Can you work these out from the model? Positions are in its coordinate system, mm. Face numbers are marked on the shaded views. A direction names the side the tool comes from. Give positions to 0.01 mm unless a question says otherwise; leave off trailing zeros. Loops run counter-clockwise (first coordinate to the right, second up) from the corner with the lowest first, then second, coordinate; pieces in that order, holes last. Notation, with made-up numbers: (74.5, 66.5) - (89.5, 66.5) arc R16 ccw to (89.5, 92.5) - close; hole circle Ø4 at (20, 23). An arc over 180 degrees is marked (long way). Answer as a JSON object with one key per item and string values. Group by question number.
Item 1: Thinking about a two-plate mould opening in X: for the marked faces 6, 7 and 8, which applies, pulls with the +X half, pulls with the -X half, needs draft (parallel to the pull), parting line crosses it, or undercut?
Item 2: Please list where these lines run through material, in increasing order: L1, parallel to X at y = 7.5, z = 3; L2, parallel to X at y = 11.5, z = -4; L3, parallel to Y at x = -13.5, z = 2.75.
Item 3: Suppose I cut it at A-A on z = 0. Count the separate pieces of the cut face and the enclosed holes in it, and give its area (3 significant figures).
Item 4: Suppose I cut it at B-B on y = 8.5. Write out the boundary of the cut face in (x, z), and give its area (3 significant figures).
Item 5: Which directions (+Z, -Z, +X, -X, +Y, -Y) give clear straight access to the entire face, cutting with the end or side of a thin tool? Please do the marked faces 1, 2, 3, 4 and 5.
Item 6: Will these pins go through, and if not, where does the flat tip stop? pin 1 (3.5 mm diameter, centred on x = 27.24, z = 0, fed in from -Y); pin 2 (3 mm diameter, centred on y = 6.5, z = -1.5, fed in from +X); pin 3 (3 mm diameter, centred on y = 6.5, z = 0, fed in from -X).
Item 7: Suppose I cut it at C-C on x = 26.5. Write out the boundary of the cut face in (y, z).
from build123d import *

# Parameters (mm, degrees)
BOSS_EXTRUDE1_DEPTH = 4.7625
FILLET1_R           = 1.5875
FILLET2_R           = 3.175
FILLET3_R           = 3.175
HOLE1_D             = 2.8448
HOLE2_D             = 2.8448


with BuildPart() as part:
    # Sketch1 → Boss-Extrude1 (new body, symmetric)
    with BuildSketch(Plane.XY):
        Polygon((-29.1465, 11.1125), (-16.764, 11.1125), (-16.764, 0), (16.764, 0), (16.764, 11.1125), (37.9095, 11.1125), (37.9095, 12.7), (15.1765, 12.7), (15.1765, 1.5875), (-15.1765, 1.5875), (-15.1765, 12.7), (-29.1465, 12.7), align=None)
    extrude(amount=BOSS_EXTRUDE1_DEPTH, both=True)

    # Fillet1
    fillet1_edges = [part.edges().sort_by_distance(p)[0] for p in [
        (-15.1765, 1.5875, 0),
        (15.1765, 1.5875, 0),
        (16.764, 11.1125, 0),
        (-16.764, 11.1125, 0),
    ]]
    fillet(fillet1_edges, radius=FILLET1_R)

    # Fillet2
    fillet2_edges = [part.edges().sort_by_distance(p)[0] for p in [
        (-15.1765, 12.7, 0),
        (15.1765, 12.7, 0),
        (16.764, 0, 0),
        (-16.764, 0, 0),
    ]]
    fillet(fillet2_edges, radius=FILLET2_R)

    # Fillet3
    fillet3_edges = [part.edges().sort_by_distance(p)[0] for p in [
        (37.9095, 11.90625, -4.7625),
        (-29.1465, 11.90625, -4.7625),
        (37.9095, 11.90625, 4.7625),
        (-29.1465, 11.90625, 4.7625),
    ]]
    fillet(fillet3_edges, radius=FILLET3_R)

    # Hole1 (through all)
    with Locations(Plane.XZ.offset(-11.1125)):
        with Locations((27.2415, 0)):
            Hole(HOLE1_D / 2)

    # Hole2 (through all)
    with Locations(Plane.XZ.offset(-11.1125)):
        with Locations((-23.5585, 0)):
            Hole(HOLE2_D / 2)


solid = part.part
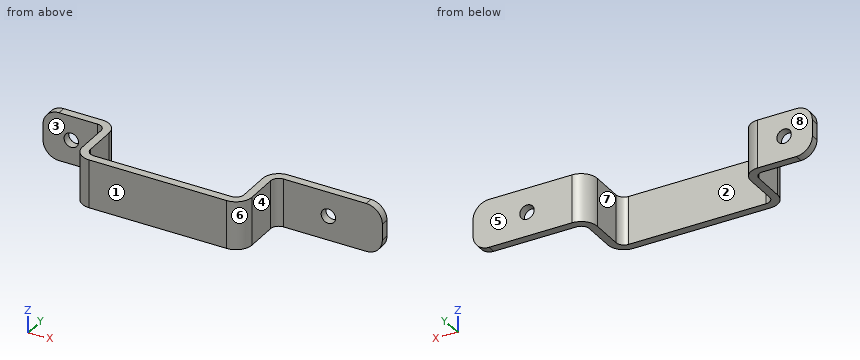
Worked out:
{
 "1": {"face 6": "pulls with the +X half", "face 7": "undercut", "face 8": "needs draft"},
 "2": {"L1": "x = -16.76 to -15.18, 15.18 to 16.76", "L2": "x = -28.04 to -15.87, 15.87 to 36.8", "L3": "y = 0 to 1.59"},
 "3": {"separate pieces": "3", "enclosed holes": "0", "area": "126 mm2"},
 "4": {"outline": "(-16.76, -4.76) - (-15.18, -4.76) - (-15.18, 4.76) - (-16.76, 4.76) - close; (15.18, -4.76) - (16.76, -4.76) - (16.76, 4.76) - (15.18, 4.76) - close", "area": "30.2 mm2"},
 "5": {"face 1": "+Z, -Z, +X, -X, -Y", "face 2": "+Z, -Z, +Y", "face 3": "+Z, -Z, -X, -Y", "face 4": "+Z, -Z, +X, -Y", "face 5": "+Z, -Z, +X, -X, +Y"},
 "6": {"pin 1": "stops at y = 11.11", "pin 2": "stops at x = 16.76", "pin 3": "stops at x = -16.76"},
 "7": {"outline": "(11.11, -4.76) - (12.7, -4.76) - (12.7, -1.21) - (11.11, -1.21) - close; (11.11, 1.21) - (12.7, 1.21) - (12.7, 4.76) - (11.11, 4.76) - close"}
}
